Model file for the job. Use its own axes, mm. A direction names the side the tool comes from. Give positions to 0.01 mm unless a question says otherwise; leave off trailing zeros. Order: outer loops, then holes, each group sorted by start corner. A loop starts at its lowest first (then second) coordinate and runs counter-clockwise, first axis right, second up. Notation, with made-up numbers: (83.5, -2) - (100.5, -2) arc R36 cw to (100.5, 32) - close; hole circle Ø11 at (-14, -38.75). An arc over 180 degrees is marked (long way). Use CSV: the item, a comma, the result in double quotes. Start each with the question number.
(1) Band-saw the part on D-D, the plane y = 54.5. Give the cut face in (x, z), then the cut area to 3 significant figures.
(2) Band-saw the part on A-A, the plane y = 0. Give the cut face in (x, z).
(3) Band-saw the part on B-B, the plane x = 0. Give the cut face in (y, z).
(4) Pull direction Y, two halves, no side cores. Call faces 4 (the flat face through (-23, 23, 4)), 5 (the flat face through (-36.922, 45.407, 1.972)), 6 (the flat face through (-30.3, -2.3, 2)), 7 (the flat face through (-45.833, 37.348, 1.972)): +Y half, -Y half, draft (parallel to the pull), parting line (faces both ways), or undercut.
(5) Tool access for faces 1 (the cylindrical face through (-34.86, 13.82, 1.97)), 2 (the cylindrical face through (-35, 33.2, 2)), 3 (the cylindrical face through (-13.58, 34.955, 1.972)): list every direction of +Z, -Z, +X, -X, +Y, -Y with a clear straight run to the whole face (end or side of a thin tool).
(6) Band-saw the part on C-C, the plane z = 1.9. Give the cut face in (x, y), then the cut area to 3 significant figures.
(7) Drop flat-ended pins along their axis: pin 1 Ø2 at (y, z) = (24.5, 3.5) entering from -X; pin 2 Ø3.5 at (x, y) = (0, 25) entering from -Z; pin 3 Ø2 at (y, z) = (10.5, 0.5) entering from -X. Give the stop position or say it passes through.
(8) Probe L1, parallel to Y at x = -25, z = 2.05; L2, parallel to Y at x = -48.5, z = 0.2; L3, parallel to X at y = 23, z = 2.7. List the from-to ranges inside material, lowest first.
from build123d import *

# Parameters (mm, degrees)
SKETCH2_R           = 3.05
SKETCH2_R_2         = 1.5
BOSS_EXTRUDE1_DEPTH = 4


with BuildPart() as part:
    # Sketch2 → Boss-Extrude1 (new body)
    with BuildSketch(Plane.XY):
        with BuildLine():
            Line((-23.142573846, -9.456282345), (9.456282345, 23.142573846))
            Line((9.456282345, 23.142573846), (-4.615964413, 37.214820603))
            ThreePointArc((-4.615964413, 37.214820603), (-13.702289069, 34.906980309), (-21.932251863, 30.417533237))
            Line((-21.932251863, 30.417533237), (-52.337843454, 60.823124828))
            Line((-52.337843454, 60.823124828), (-60.823124828, 52.337843454))
            Line((-60.823124828, 52.337843454), (-30.417533237, 21.932251863))
            ThreePointArc((-30.417533237, 21.932251863), (-34.906980309, 13.702289069), (-37.214820603, 4.615964413))
            Line((-37.214820603, 4.615964413), (-23.142573846, -9.456282345))
        make_face()
        with Locations((0, 25)):
            Circle(SKETCH2_R, mode=Mode.SUBTRACT)
        with Locations((-25, 0)):
            Circle(SKETCH2_R, mode=Mode.SUBTRACT)
        with Locations((-48.802309548, 48.802309548)):
            Circle(SKETCH2_R_2, mode=Mode.SUBTRACT)
        with Locations((-34.660173924, 34.660173924)):
            Circle(SKETCH2_R_2, mode=Mode.SUBTRACT)
    extrude(amount=BOSS_EXTRUDE1_DEPTH)


solid = part.part
Answer block:
1,outline,"(-58.66, 0) - (-46.01, 0) - (-46.01, 4) - (-58.66, 4) - close"
1,area,"50.6 mm2"
2,outline,"(-32.6, 0) - (-28.05, 0) - (-28.05, 4) - (-32.6, 4) - close; (-21.95, 0) - (-13.69, 0) - (-13.69, 4) - (-21.95, 4) - close"
3,outline,"(13.69, 0) - (21.95, 0) - (21.95, 4) - (13.69, 4) - close; (28.05, 0) - (32.6, 0) - (32.6, 4) - (28.05, 4) - close"
4,face 4,"draft"
4,face 5,"+Y half"
4,face 6,"-Y half"
4,face 7,"undercut"
5,face 1,"+Z, -Z, -X"
5,face 2,"+Z, -Z"
5,face 3,"+Z, -Z, +Y"
6,outline,"(-60.82, 52.34) - (-30.42, 21.93) arc R37.5 ccw to (-37.21, 4.62) - (-23.14, -9.46) - (9.46, 23.14) - (-4.62, 37.21) arc R37.5 ccw to (-21.93, 30.42) - (-52.34, 60.82) - close; hole circle Ø3 at (-48.8, 48.8); hole circle Ø3 at (-34.66, 34.66); hole circle Ø6.1 at (-25, 0); hole circle Ø6.1 at (0, 25)"
6,area,"1,610 mm2"
7,pin 1,"stops at x = -33.99"
7,pin 2,"passes through"
7,pin 3,"stops at x = -36.28"
8,L1,"y = -7.6 to -3.05, 3.05 to 33.49"
8,L2,"y = 40.01 to 47.33, 50.27 to 56.99"
8,L3,"x = -31.49 to -2.3, 2.3 to 9.31"
